from build123d import *

# Parameters (mm, degrees)
F0_R     = 19.5
F1_DEPTH = 30
F2_SIZE  = 1
F5_R     = 15.25
F6_DEPTH = 30
F7_W     = 0.5
F7_H     = 0.5
F8_DEPTH = 29.032


with BuildPart() as f1:
    # F0 (on Top) → F1 (new body)
    with BuildSketch(Plane.XY):
        Circle(F0_R)
    extrude(amount=-F1_DEPTH)

    # F2
    f2_edges = [f1.edges().sort_by_distance(p)[0] for p in [
        (-19.5, 0, 0),
    ]]
    chamfer(f2_edges, length=F2_SIZE)

    # F3 (on Front) → F4 (revolve)
    with BuildSketch(Plane.XZ):
        Polygon((19.25, -30), (0, -30), (0, -39), (17.6423, -39), align=None)
    revolve(axis=Axis((0, 0, -34.5), (0, 0, -1)))

    # F5 (on face) → F6 (cut)
    with BuildSketch(Plane(origin=(0, 0, -39), x_dir=(1, 0, 0), z_dir=(0, 0, -1))):
        with Locations((0.772339, 0)):
            Circle(F5_R)
    extrude(amount=-F6_DEPTH, mode=Mode.SUBTRACT)

    # F7 (on face) → F8 (cut)
    with BuildSketch(Plane.XY):
        with Locations((0, 19.501211)):
            Rectangle(F7_W, F7_H)
        Polygon((-4.351045, 19.267622), (-4.247089, 18.778548), (-3.758015, 18.882504), (-3.861971, 19.371578), align=None)
        Polygon((-8.261928, 17.941945), (-8.058559, 17.485172), (-7.601787, 17.688541), (-7.805155, 18.145313), align=None)
        Polygon((-11.811725, 15.832119), (-11.517832, 15.427611), (-11.113324, 15.721503), (-11.407216, 16.126012), align=None)
        Polygon((-14.845293, 13.030354), (-14.473721, 12.695788), (-14.139155, 13.067361), (-14.510728, 13.401926), align=None)
        Polygon((-17.230051, 9.659099), (-16.797038, 9.409099), (-16.547038, 9.842112), (-16.980051, 10.092112), align=None)
        Polygon((-18.861772, 5.865696), (-18.386244, 5.711187), (-18.231736, 6.186716), (-18.707264, 6.341224), align=None)
        Polygon((-19.669144, 1.815933), (-19.171883, 1.763669), (-19.119619, 2.26093), (-19.61688, 2.313194), align=None)
        Polygon((-19.61688, -2.313194), (-19.119619, -2.26093), (-19.171883, -1.763669), (-19.669144, -1.815933), align=None)
        Polygon((-18.707264, -6.341224), (-18.231736, -6.186716), (-18.386244, -5.711187), (-18.861772, -5.865696), align=None)
        Polygon((-16.980051, -10.092112), (-16.547038, -9.842112), (-16.797038, -9.409099), (-17.230051, -9.659099), align=None)
        Polygon((-14.510728, -13.401926), (-14.139155, -13.067361), (-14.473721, -12.695788), (-14.845293, -13.030354), align=None)
        Polygon((-11.407216, -16.126012), (-11.113324, -15.721503), (-11.517832, -15.427611), (-11.811725, -15.832119), align=None)
        Polygon((-7.805155, -18.145313), (-7.601787, -17.688541), (-8.058559, -17.485172), (-8.261928, -17.941945), align=None)
        Polygon((-3.861971, -19.371578), (-3.758015, -18.882504), (-4.247089, -18.778548), (-4.351045, -19.267622), align=None)
        with Locations((0, -19.501211)):
            Rectangle(F7_W, F7_H)
        Polygon((4.351045, -19.267622), (4.247089, -18.778548), (3.758015, -18.882504), (3.861971, -19.371578), align=None)
        Polygon((8.261928, -17.941945), (8.058559, -17.485172), (7.601787, -17.688541), (7.805155, -18.145313), align=None)
        Polygon((11.811725, -15.832119), (11.517832, -15.427611), (11.113324, -15.721503), (11.407216, -16.126012), align=None)
        Polygon((14.845293, -13.030354), (14.473721, -12.695788), (14.139155, -13.067361), (14.510728, -13.401926), align=None)
        Polygon((17.230051, -9.659099), (16.797038, -9.409099), (16.547038, -9.842112), (16.980051, -10.092112), align=None)
        Polygon((18.861772, -5.865696), (18.386244, -5.711187), (18.231736, -6.186716), (18.707264, -6.341224), align=None)
        Polygon((19.669144, -1.815933), (19.171883, -1.763669), (19.119619, -2.26093), (19.61688, -2.313194), align=None)
        Polygon((19.61688, 2.313194), (19.119619, 2.26093), (19.171883, 1.763669), (19.669144, 1.815933), align=None)
        Polygon((18.707264, 6.341224), (18.231736, 6.186716), (18.386244, 5.711187), (18.861772, 5.865696), align=None)
        Polygon((16.980051, 10.092112), (16.547038, 9.842112), (16.797038, 9.409099), (17.230051, 9.659099), align=None)
        Polygon((14.510728, 13.401926), (14.139155, 13.067361), (14.473721, 12.695788), (14.845293, 13.030354), align=None)
        Polygon((11.407216, 16.126012), (11.113324, 15.721503), (11.517832, 15.427611), (11.811725, 15.832119), align=None)
        Polygon((7.805155, 18.145313), (7.601787, 17.688541), (8.058559, 17.485172), (8.261928, 17.941945), align=None)
        Polygon((3.861971, 19.371578), (3.758015, 18.882504), (4.247089, 18.778548), (4.351045, 19.267622), align=None)
    extrude(amount=-F8_DEPTH, mode=Mode.SUBTRACT)


solid = f1.part
CAD build for the part. Positions are in the model's coordinates, mm. A direction names the side the tool comes from. Round coordinates to 2 decimals unless told otherwise and drop trailing zeros. Write each loop counter-clockwise with the first axis right and the second up, starting at its lowest first coordinate (ties: lowest second). Pieces come first, ordered by that corner, then holes. Notation, with made-up numbers: M 31.5,57 L 52.5,57 A13 ccw 52.5,72 Z; hole C 21,49 d1. An arc over 180 degrees is marked long. Put each result on its own line as item: value. Start each with the question number.
1) Pin check, flat tips, straight feed: pin 1 Ø10 at (x, z) = (7, -18.5) entering from -Y; pin 2 Ø12 at (x, z) = (-14, -15.5) entering from +Y; pin 3 Ø8 at (x, z) = (9.5, -16.5) entering from +Y. Stop position of each tip, or through.
2) Pull direction X, two halves, no side cores. Call faces 1 (the conical face through (-2.33, -17.77, -37.44)), 2 (the flat face through (-13, -7, -39)), 3 (the flat face through (1, 0, -9)): pulls with the +X half, pulls with the -X half, needs draft (parallel to the pull), parting line crosses it, or undercut.
3) 3-axis set-ups, long thin cutter, end or side, ignore diameter. For faces 4 (the cylindrical face through (-2.53, 14.89, -24.21)), 5 (the flat face through (0, 0, 0)): which of +Z, -Z, +X, -X, +Y, -Y reach the whole face in a straight line?
4) Drill centre lines: probe 1 along X at (y, z) = (0, -25); probe 2 along X at (y, z) = (-15.5, -10.5); probe 3 along Z at (x, y) = (13, 4.5). Where is each one in solid material? Low to high. Write a range as [from, to].
5) Saw through at A-A, the plane y = 0. Write the cut outline in (x, z), and give its area (3 significant figures).
6) Saw through at B-B, the plane z = -34.5. Write the cut outline in (x, y).
Resolved:
1. pin 1: y = -19.4
1. pin 2: y = 17.71
1. pin 3: y = 18.71
2. face 1: parting line crosses it
2. face 2: needs draft
2. face 3: undercut
3. face 4: -Z
3. face 5: +Z, +X, -X, +Y, -Y
4. probe 1: [-19.5, -14.48], [16.02, 19.5]
4. probe 2: [-11.83, -11.57], [-11.42, 11.42], [11.57, 11.83]
4. probe 3: [-9, 0]
5. outline: M -19.5,-30 L -19.25,-30 L -17.64,-39 L -14.48,-39 L -14.48,-9 L 16.02,-9 L 16.02,-39 L 17.64,-39 L 19.25,-30 L 19.5,-30 L 19.5,-1 L 18.5,0 L -18.5,0 L -19.5,-1 Z
5. area: 586 mm²
6. outline: C 0,0 d36.89; hole C 0.77,0 d30.5
